Verification items for the finished model (mm, model axes). A direction names the side the tool comes from. Give positions to 0.01 mm unless a question says otherwise; leave off trailing zeros. Write each loop counter-clockwise with the first axis right and the second up, starting at its lowest first coordinate (ties: lowest second). Pieces come first, ordered by that corner, then holes. Notation, with made-up numbers: (72.25, -37) -> (83.25, -37) arc R19 ccw to (83.25, -13) -> close; hole circle Ø7 at (-29, -11.5). An arc over 180 degrees is marked (long way). Use one line per item in the form item = value. Start each with the question number.
(1) Section check C-C, the plane y = 0. Record the cut outline in (x, z), plus the area to 3 significant figures.
(2) Release check for a two-part mould opening along Y. For faces 1 (the face through (38, -8, 9)), 2 (the face through (-30, 17.6, 3)), 3 (the face through (36, 0, 6)) record: pulls with the +Y half, pulls with the -Y half, needs draft (parallel to the pull), parting line crosses it, or undercut.
(3) Scan lines: L1, parallel to Y at x = 0, z = 5.25; L2, parallel to Y at x = 41, z = 7.75; L3, parallel to X at y = 1, z = 17. Record each from-to range of solid material in increasing order.
(4) Section check B-B, the plane x = -41. Record the cut outline in (y, z).
(5) Set-up check for faces 4 (the face through (-33, 13, 6)), 5 (the face through (32, -13, 6)), 6 (the face through (38, 8, 9)): record each of +Z, -Z, +X, -X, +Y, -Y from which the full face is reachable in a straight line by a thin tool's end or side.
(6) Section check D-D, the plane x = 0. Record the cut outline in (y, z), plus the area to 3 significant figures.
(7) Depth check by flat-ended pin: pin 1 Ø5.5 at (x, y) = (37, 13) entering from +Z; pin 2 Ø4 at (x, z) = (19.5, 14) entering from +Y; pin 3 Ø5 at (x, y) = (41, -3) entering from +Z; pin 4 Ø6 at (x, y) = (0, -50) entering from +Z. Enter the tip coordinate at first touch or a pass-through.
(8) Section check A-A, the plane z = 10.25. Record the cut outline in (x, y), plus the area to 3 significant figures.
from build123d import *

# Parameters (mm, degrees)
SKETCH1_R             = 5
BOSS_EXTRUDE1_DEPTH   = 12
BOSS_EXTRUDE1_2_DEPTH = 12
BOSS_EXTRUDE1_3_DEPTH = 12
BOSS_EXTRUDE2_DEPTH   = 6
SKETCH1_4_R           = 30
SKETCH1_4_R_2         = 25
BOSS_EXTRUDE3_DEPTH   = 30


with BuildPart() as part:
    # Sketch1 → Boss-Extrude1 (new body)
    with BuildSketch(Plane.XY):
        with BuildLine():
            ThreePointArc((-28.91366459, -8), (-30, 0), (-28.91366459, 8))
            Line((-28.91366459, 8), (-47, 8))
            ThreePointArc((-47, 8), (-51, 0), (-47, -8))
            Line((-47, -8), (-28.91366459, -8))
        make_face()
        with Locations((-41, 0)):
            Circle(SKETCH1_R, mode=Mode.SUBTRACT)
    extrude(amount=BOSS_EXTRUDE1_DEPTH)



with BuildPart() as body_2:
    # Sketch1 → Boss-Extrude1 2 (new body)
    with BuildSketch(Plane.XY):
        with BuildLine():
            ThreePointArc((47, -8), (51, 0), (47, 8))
            Line((47, 8), (28.91366459, 8))
            ThreePointArc((28.91366459, 8), (29.727175595, 4.036710437), (30, 0))
            ThreePointArc((30, 0), (29.727175595, -4.036710437), (28.91366459, -8))
            Line((28.91366459, -8), (47, -8))
        make_face()
        with Locations((41, 0)):
            Circle(SKETCH1_R, mode=Mode.SUBTRACT)
    extrude(amount=BOSS_EXTRUDE1_2_DEPTH)


with BuildPart() as body_3:
    # Sketch1 → Boss-Extrude1 3 (new body)
    with BuildSketch(Plane.XY):
        with BuildLine():
            Line((23.454044644, -21.260032532), (27.49545417, -12))
            ThreePointArc((27.49545417, -12), (0, -30), (-27.49545417, -12))
            Line((-27.49545417, -12), (-23.454044644, -21.260032532))
            Line((-23.454044644, -21.260032532), (-9.16515139, -54))
            ThreePointArc((-9.16515139, -54), (0, -60), (9.16515139, -54))
            Line((9.16515139, -54), (23.454044644, -21.260032532))
        make_face()
        with Locations((0, -50)):
            Circle(SKETCH1_R, mode=Mode.SUBTRACT)
    extrude(amount=BOSS_EXTRUDE1_3_DEPTH)


with BuildPart() as part_1:
    add(part.part)

    add(body_2.part)  # Boss-Extrude2 merges body 2

    add(body_3.part)  # Boss-Extrude2 merges body 3
    # Sketch1_3 → Boss-Extrude2 (add)
    with BuildSketch(Plane.XY):
        with BuildLine():
            ThreePointArc((-27.49545417, -12), (-28.275380984, -10.025109984), (-28.91366459, -8))
            Line((-28.91366459, -8), (-47, -8))
            ThreePointArc((-47, -8), (-46.451241941, -8.383553024), (-45.87804878, -8.729526911))
            Line((-45.87804878, -8.729526911), (-23.454044644, -21.260032532))
            Line((-23.454044644, -21.260032532), (-27.49545417, -12))
        make_face()
        with BuildLine():
            ThreePointArc((-28.91366459, 8), (-23.596802252, 18.52541291), (-14.634146341, 26.188580734))
            Line((-14.634146341, 26.188580734), (-45.87804878, 8.729526911))
            ThreePointArc((-45.87804878, 8.729526911), (-46.451241941, 8.383553024), (-47, 8))
            Line((-47, 8), (-28.91366459, 8))
        make_face()
        with BuildLine():
            ThreePointArc((47, 8), (46.451241941, 8.383553024), (45.87804878, 8.729526911))
            Line((45.87804878, 8.729526911), (14.634146341, 26.188580734))
            ThreePointArc((14.634146341, 26.188580734), (23.596802252, 18.52541291), (28.91366459, 8))
            Line((28.91366459, 8), (47, 8))
        make_face()
        with BuildLine():
            ThreePointArc((45.87804878, -8.729526911), (46.451241941, -8.383553024), (47, -8))
            Line((47, -8), (28.91366459, -8))
            ThreePointArc((28.91366459, -8), (28.275380984, -10.025109984), (27.49545417, -12))
            Line((27.49545417, -12), (23.454044644, -21.260032532))
            Line((23.454044644, -21.260032532), (45.87804878, -8.729526911))
        make_face()
    extrude(amount=BOSS_EXTRUDE2_DEPTH)

    # Sketch1_4 → Boss-Extrude3 (add)
    with BuildSketch(Plane.XY):
        with Locations(Location((0, 0, 0), (0, 0, 164.533990047))):
            Circle(SKETCH1_4_R)
        Circle(SKETCH1_4_R_2, mode=Mode.SUBTRACT)
    extrude(amount=BOSS_EXTRUDE3_DEPTH)


solid = part_1.part
Completed:
q1.outline = (-51, 0) -> (-46, 0) -> (-46, 12) -> (-51, 12) -> close; (-36, 0) -> (-25, 0) -> (-25, 30) -> (-30, 30) -> (-30, 12) -> (-36, 12) -> close; (25, 0) -> (36, 0) -> (36, 12) -> (30, 12) -> (30, 30) -> (25, 30) -> close; (46, 0) -> (51, 0) -> (51, 12) -> (46, 12) -> close
q1.area = 564 mm²
q2.face_1 = pulls with the -Y half
q2.face_2 = pulls with the +Y half
q2.face_3 = undercut
q3.L1 = -60 to -55, -45 to -25, 25 to 30
q3.L2 = -8 to -5, 5 to 8
q3.L3 = -29.98 to -24.98, 24.98 to 29.98
q4.outline = (-11.46, 0) -> (-5, 0) -> (-5, 12) -> (-8, 12) -> (-8, 6) -> (-11.46, 6) -> close; (5, 0) -> (11.46, 0) -> (11.46, 6) -> (8, 6) -> (8, 12) -> (5, 12) -> close
q5.face_4 = +Z, -X, +Y
q5.face_5 = +Z, +X, -Y
q5.face_6 = +Z, +X, +Y
q6.outline = (-60, 0) -> (-55, 0) -> (-55, 12) -> (-60, 12) -> close; (-45, 0) -> (-25, 0) -> (-25, 30) -> (-30, 30) -> (-30, 12) -> (-45, 12) -> close; (25, 0) -> (30, 0) -> (30, 30) -> (25, 30) -> close
q6.area = 540 mm²
q7.pin_1 = 6
q7.pin_2 = 24.37
q7.pin_3 = 12
q7.pin_4 = through
q8.outline = (-47, -8) -> (-28.91, -8) arc R30 ccw to (-27.5, -12) -> (-9.17, -54) arc R10 ccw to (9.17, -54) -> (27.5, -12) arc R30 ccw to (28.91, -8) -> (47, -8) arc R10 ccw to (47, 8) -> (28.91, 8) arc R30 ccw to (-28.91, 8) -> (-47, 8) arc R10 ccw to start; hole circle Ø10 at (-41, 0); hole circle Ø50 at (0, 0); hole circle Ø10 at (0, -50); hole circle Ø10 at (41, 0)
q8.area = 2,180 mm²
